Geometry check sheet. Reference: drawing and pictorial views, mm from the part's lowest x, y, z. Round coordinates to 2 decimals unless told otherwise and drop trailing zeros. Order: outer loops, then holes, each group sorted by start corner. A loop starts at its lowest first (then second) coordinate and runs counter-clockwise, first axis right, second up.
Q1. Cross-section at A-A on y = 12.8. Record the cut outline in (x, z), then the cut area to 3 significant figures.
Q2. Cross-section at C-C on z = 36. Record the cut outline in (x, y).
Q3. Depth check by flat-ended pin: P1, Ø1.8, axis at x = 12.5, y = 14, coming from the -Z side; P2, Ø8, axis at y = 17.5, z = 17, coming from the -X side; P3, Ø1.5, axis at y = 10.5, z = 35, coming from the +X side. Enter the tip coordinate at first touch or a pass-through.
Q4. Mould release check, pull along Y, two halves, no side actions. Record for the marked faces 1, 2 and 3: +Y half, -Y half, draft (parallel to the pull), parting line (faces both ways), or undercut.
Q5. Scan lines: probe 1 along Y at (x, z) = (12.8, 2.25); probe 2 along Z at (x, y) = (11, 13.5); probe 3 along X at (y, z) = (19, 35). Record each from-to range of solid material in increasing order.
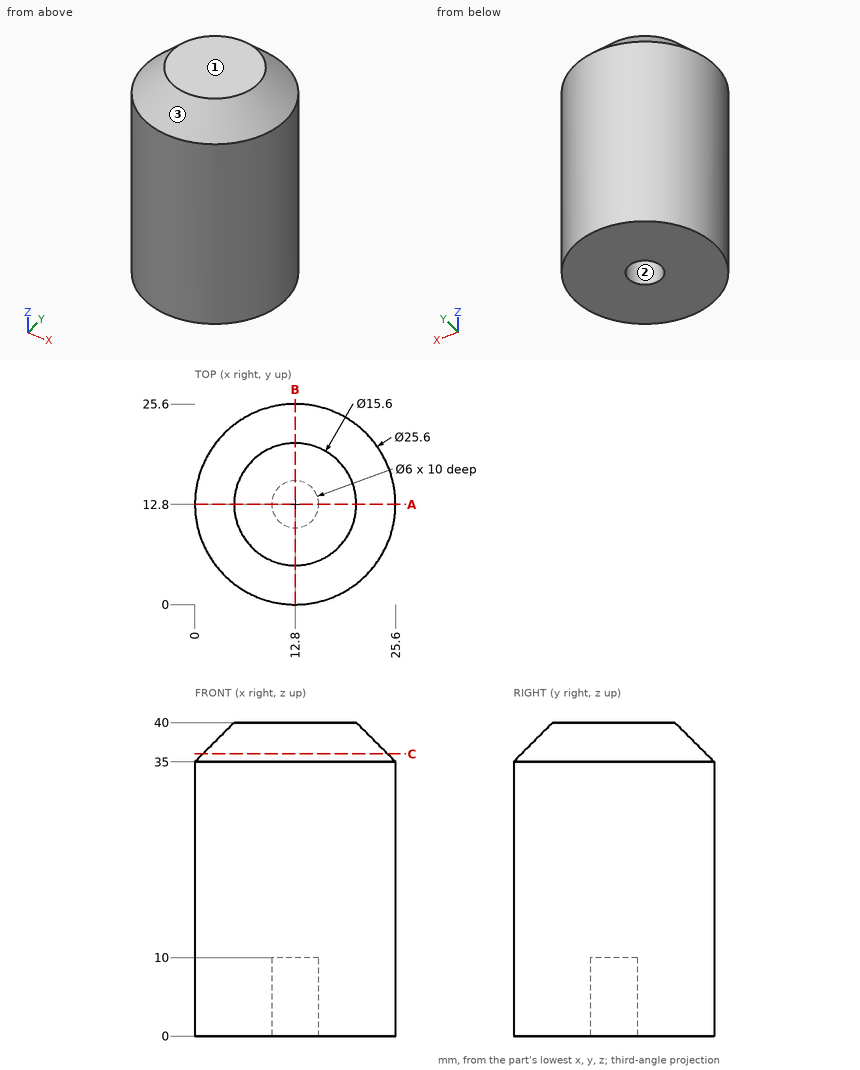
Results found:
1. outline: (0, 0) - (9.8, 0) - (9.8, 10) - (15.8, 10) - (15.8, 0) - (25.6, 0) - (25.6, 35) - (20.6, 40) - (5, 40) - (0, 35) - close
1. area: 939 mm2
2. outline: circle Ø23.6 at (12.8, 12.8)
3. P1: stops at z = 10
3. P2: stops at x = 0.02
3. P3: stops at x = 25.51
4. face 1: draft
4. face 2: undercut
4. face 3: parting line
5. probe 1: y = 0 to 9.8, 15.8 to 25.6
5. probe 2: z = 10 to 40
5. probe 3: x = 1.6 to 24
